from build123d import *

# Parameters (mm, degrees)
SKETCH1_R              = 43.18
FLANGE_EXTRUDE_DEPTH   = 12.7
SKETCH2_R              = 15.0876
AN_FITTING_BODY_DEPTH  = 23.114
HOLE_FOR_FITTING_REACH = 37.814
SKETCH3_R              = 10.668
SKETCH5_R              = 16.637
SKETCH5_R_2            = 15.0876
MEAT_FOR_THREAD_DEPTH  = 11.7094
SKETCH10_R             = 15.1892
SKETCH10_R_2           = 12.7
O_RING_GROOVE_DEPTH    = 1.26238
SKETCH13_R             = 3.175
BOLT_HOLE_DEPTH        = 12.7
CIRPATTERN1_COUNT      = 8


with BuildPart() as part:
    # Sketch1 → flange extrude (new body)
    with BuildSketch(Plane(origin=(0, 0, 0), x_dir=(1, 0, 0), z_dir=(0, 1, 0))):
        Circle(SKETCH1_R)
    extrude(amount=FLANGE_EXTRUDE_DEPTH)

    # Sketch2 → an fitting body (add)
    with BuildSketch(Plane(origin=(0, 12.7, 0), x_dir=(1, 0, 0), z_dir=(0, 1, 0))):
        Circle(SKETCH2_R)
    extrude(amount=AN_FITTING_BODY_DEPTH)

    # Sketch3 → hole for fitting (cut, up to next)
    with BuildSketch(Plane(origin=(0, 35.814, 0), x_dir=(1, 0, 0), z_dir=(0, 1, 0)), mode=Mode.PRIVATE) as hole_for_fitting_sk1:
        Circle(SKETCH3_R)
    hole_for_fitting_tool1 = extrude(hole_for_fitting_sk1.sketch, amount=-HOLE_FOR_FITTING_REACH, mode=Mode.PRIVATE) & part.part
    add(hole_for_fitting_tool1.solids().sort_by_distance((0, 35.814, 0))[0], mode=Mode.SUBTRACT)

    # Sketch5 → meat for thread (add)
    with BuildSketch(Plane(origin=(0, 16.1798, 0), x_dir=(1, 0, 0), z_dir=(0, 1, 0))):
        Circle(SKETCH5_R)
        Circle(SKETCH5_R_2, mode=Mode.SUBTRACT)
    extrude(amount=MEAT_FOR_THREAD_DEPTH)

    # Sketch6 → Cut-Revolve1 (revolve, cut)
    with BuildSketch(Plane.XY):
        Polygon((12.6873, 35.814), (15.0876, 32.628694315), (15.0876, 35.814), align=None)
    revolve(axis=Axis((0, 0, 0), (0, 1, 0)), mode=Mode.SUBTRACT)

    # Sketch10 → O-ring groove (cut)
    with BuildSketch(Plane.XZ):
        Circle(SKETCH10_R)
        Circle(SKETCH10_R_2, mode=Mode.SUBTRACT)
    extrude(amount=-O_RING_GROOVE_DEPTH, mode=Mode.SUBTRACT)

    # Sketch13 → bolt hole (cut)
    with BuildSketch(Plane.XZ):
        with Locations((0, 31.75)):
            Circle(SKETCH13_R)
    bolt_hole = extrude(amount=-BOLT_HOLE_DEPTH, mode=Mode.SUBTRACT)

    # CirPattern1: bolt hole ×8 about axis
    cirpattern1_axis = Axis((0, 0, 0), (0, 1, 0))
    for i in range(1, CIRPATTERN1_COUNT):
        add(bolt_hole.rotate(cirpattern1_axis, i * 360 / CIRPATTERN1_COUNT), mode=Mode.SUBTRACT)


solid = part.part
Model file for the job. Use its own axes, mm. A direction names the side the tool comes from. Give positions to 0.01 mm unless a question says otherwise; leave off trailing zeros. Order: outer loops, then holes, each group sorted by start corner. A loop starts at its lowest first (then second) coordinate and runs counter-clockwise, first axis right, second up. Notation, with made-up numbers: (56, -33) - (73, -33) arc R11 ccw to (73, -17) - close; hole circle Ø10 at (80, 68.5). An arc over 180 degrees is marked (long way). Return JSON: item names as keys, results as strings.
1) Cut at A-A, the plane z = 0. Count the separate pieces of the cut face and the enclosed holes in it, plus the area to 3 significant figures.
Geometry says:
{"separate pieces": "4", "enclosed holes": "0", "area": "891 mm²"}
2) Pull direction X, two halves, no side cores. Call faces 5 (the cylindrical face through (28.65, 6.26, 0.69)), 6 (the conical face through (-2.783, 35.615, 12.532)), 7 (the flat face through (19, 0, -1)): pulls with the +X half, pulls with the -X half, needs draft (parallel to the pull), parting line crosses it, or undercut.
Geometry says:
{"face 5": "undercut", "face 6": "parting line crosses it", "face 7": "needs draft"}
3) Flat gauge pins, fed straight in: P1, Ø6, axis at x = -34.5, z = -16, coming from the +Y side; P2, Ø2, axis at y = 31.5, z = 10.5, coming from the +X side; P3, Ø15, axis at x = 5.5, z = 7.5, coming from the -Y side; P4, Ø5.5, axis at x = -22.45, z = -22.45, coming from the +Y side. Where does each tip first touch, or does it go through?
Geometry says:
{"P1": "y = 12.7", "P2": "x = 11.72", "P3": "y = 0", "P4": "through"}
4) Cut at B-B, the plane y = 22. Give the cut face in (x, z).
Geometry says:
{"outline": "circle Ø33.27 at (0, 0); hole circle Ø21.34 at (0, 0)"}
5) 3-axis set-ups, long thin cutter, end or side, ignore diameter. For faces 1 (the flat face through (4, 16.18, 15)), 2 (the cylindrical face through (-11.973, 30.226, 9.181)), 3 (the flat face through (7, 1.262, -11)), 4 (the cylindrical face through (-0.69, 6.26, 28.65)): which of +Z, -Z, +X, -X, +Y, -Y reach the whole face in a straight line?
Geometry says:
{"face 1": "none", "face 2": "+Y", "face 3": "-Y", "face 4": "+Y, -Y"}
6) Cut at D-D, the plane z = 30.5. Give the cut face in (x, y), plus the area to 3 significant figures.
Geometry says:
{"outline": "(-30.57, 0) - (-2.92, 0) - (-2.92, 12.7) - (-30.57, 12.7) - close; (2.92, 0) - (30.57, 0) - (30.57, 12.7) - (2.92, 12.7) - close", "area": "702 mm²"}
7) Probe line 1 (Z direction, x = 0, y = 4) (3 decimals); line 2 (Y direction, x = 4.5, z = -29.5). List the from-to ranges inside material, lowest first. Write a range as from..to.
Geometry says:
{"line 1": "-43.18..-34.925, -28.575..-10.668, 10.668..28.575, 34.925..43.18", "line 2": "0..12.7"}
